Answer from the drawing. Dimensions are ordinates in mm from the lowest x, y and z of the part. A direction names the side the tool comes from. Coordinates: 2 decimals unless noted, no trailing zeros. Write each loop counter-clockwise with the first axis right and the second up, starting at its lowest first coordinate (ties: lowest second). Pieces come first, ordered by that corner, then holes. Notation, with made-up numbers: (67.5, 27.25) - (96.5, 27.25) arc R18 cw to (96.5, 51.25) - close; hole circle Ø5 at (-27, -8.5). An arc over 180 degrees is marked (long way). Use a Markdown table: item, result.
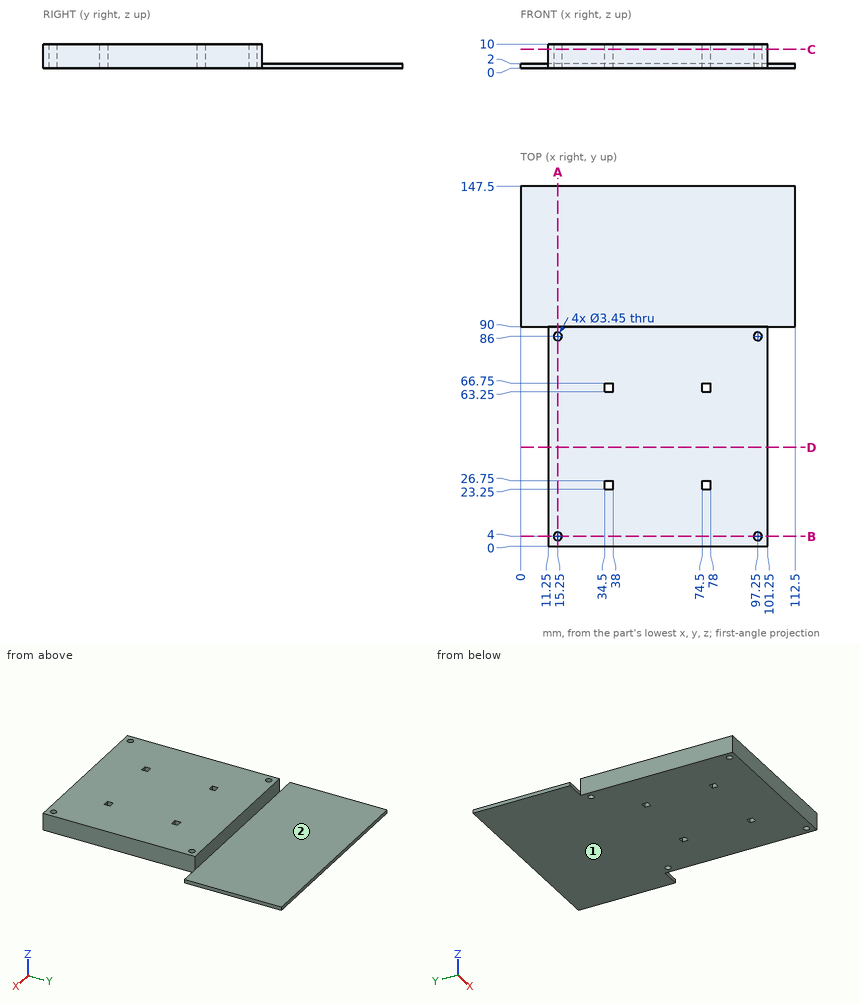
(1) A cutting plane is placed at C-C, the plane z = 7.75. Count the separate pieces of the cut face and the enclosed holes in it, and give its area (3 significant figures).
Report:
| item | result |
|---|---|
| separate pieces | 1 |
| enclosed holes | 8 |
| area | 8,010 mm² |
(2) A cutting plane is placed at B-B, the plane y = 4. Write down the section's boundary in (x, z) (3 decimals).
Report:
| item | result |
|---|---|
| outline | (11.25, 0) - (13.525, 0) - (13.525, 10) - (11.25, 10) - close; (16.975, 0) - (95.525, 0) - (95.525, 10) - (16.975, 10) - close; (98.975, 0) - (101.25, 0) - (101.25, 10) - (98.975, 10) - close |
(3) A cutting plane is placed at D-D, the plane y = 40.5. Write down the section's boundary in (x, z), and give its area (3 significant figures).
Report:
| item | result |
|---|---|
| outline | (11.25, 0) - (101.25, 0) - (101.25, 10) - (11.25, 10) - close |
| area | 900 mm² |
(4) For the marked faces 1 and 2, determine the directions among +Z, -Z, +X, -X, +Y, -Y from which every point of the face is accessible in a straight line to the end or side of a thin tool.
Report:
| item | result |
|---|---|
| face 1 | -Z, +X, -X, +Y, -Y |
| face 2 | +Z, +X, -X, +Y |
(5) Straight lines are drawn through the part: L1, parallel to Y at x = 36.5, z = 8.25; L2, parallel to Y at x = 97, z = 9; L3, parallel to X at y = 86, z = 3.25 (3 decimals). For each, find the intervals that lie inside material, in ascending order.
Report:
| item | result |
|---|---|
| L1 | y = 0 to 23.25, 26.75 to 63.25, 66.75 to 90 |
| L2 | y = 0 to 2.29, 5.71 to 84.29, 87.71 to 90 |
| L3 | x = 11.25 to 13.525, 16.975 to 95.525, 98.975 to 101.25 |
(6) Each of these flat-tipped pins is pushed along its axis until it touches: P1, Ø2, axis at y = 81.5, z = 8, coming from the -X side; P2, Ø1.6, axis at x = 106.5, z = 1, coming from the -Y side; P3, Ø1.8, axis at y = 66, z = 5, coming from the +X side; P4, Ø3, axis at x = 35.5, y = 112, coming from the -Z side. Where does it stop, or does it pass through?
Report:
| item | result |
|---|---|
| P1 | stops at x = 11.25 |
| P2 | stops at y = 90 |
| P3 | stops at x = 101.25 |
| P4 | stops at z = 0 |
(7) A cutting plane is placed at A-A, the plane x = 15.25. Write down the section's boundary in (y, z) (3 decimals).
Report:
| item | result |
|---|---|
| outline | (0, 0) - (2.275, 0) - (2.275, 10) - (0, 10) - close; (5.725, 0) - (84.275, 0) - (84.275, 10) - (5.725, 10) - close; (87.725, 0) - (147.5, 0) - (147.5, 2) - (90, 2) - (90, 10) - (87.725, 10) - close |
